Source: CAD feature listing. Evaluate the final solid. Frame: model axes, mm. Face numbers are marked on the shaded views. A direction names the side the tool comes from. Give positions to 0.01 mm unless a question says otherwise; leave off trailing zeros. Order: outer loops, then holes, each group sorted by start corner. A loop starts at its lowest first (then second) coordinate and runs counter-clockwise, first axis right, second up. Notation, with made-up numbers: (45.25, -29.75) -> (80.25, -29.75) arc R18 cw to (80.25, -7.75) -> close; hole circle Ø5 at (-9, 75.5). An arc over 180 degrees is marked (long way). Use one line per item in the form item = value. Start each with the question number.
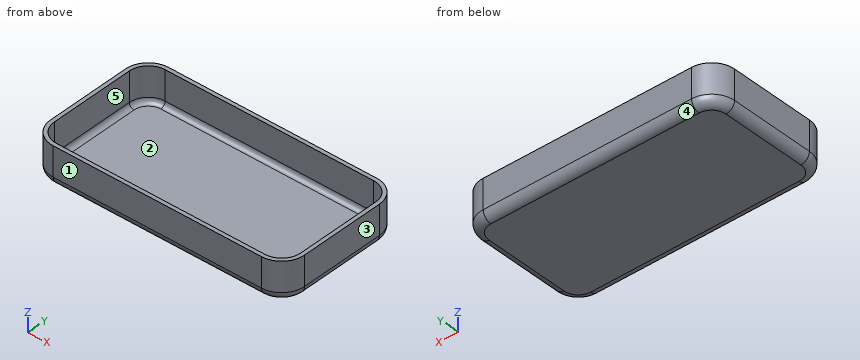
from build123d import *

# Parameters (mm, degrees)
F0_W     = 53.4
F0_H     = 27.4
F0_W_2   = 51.8
F0_H_2   = 25.8
F1_DEPTH = 0.8
F2_DEPTH = 8
F3_R     = 4
F4_R     = 4.8
F5_R     = 1
F6_R     = 1.8


with BuildPart() as f1:
    # F0 (on Top) → F1 (new body)
    with BuildSketch(Plane.XY):
        Rectangle(F0_W, F0_H)
        Rectangle(F0_W_2, F0_H_2, mode=Mode.SUBTRACT)
        Rectangle(F0_W_2, F0_H_2)
    extrude(amount=F1_DEPTH)

    # F0 (on Top) → F2 (join)
    with BuildSketch(Plane.XY):
        Rectangle(F0_W, F0_H)
        Rectangle(F0_W_2, F0_H_2, mode=Mode.SUBTRACT)
    extrude(amount=F2_DEPTH)

    # F3
    f3_edges = [f1.edges().sort_by_distance(p)[0] for p in [
        (-25.9, 12.9, 4.4),
        (25.9, 12.9, 4.4),
        (25.9, -12.9, 4.4),
        (-25.9, -12.9, 4.4),
    ]]
    fillet(f3_edges, radius=F3_R)

    # F4
    f4_edges = [f1.edges().sort_by_distance(p)[0] for p in [
        (26.7, 13.7, 4),
        (26.7, -13.7, 4),
        (-26.7, 13.7, 4),
        (-26.7, -13.7, 4),
    ]]
    fillet(f4_edges, radius=F4_R)

    # F5
    f5_edges = [f1.edges().sort_by_distance(p)[0] for p in [
        (0, 12.9, 0.8),
    ]]
    fillet(f5_edges, radius=F5_R)

    # F6
    f6_edges = [f1.edges().sort_by_distance(p)[0] for p in [
        (0, 13.7, 0),
    ]]
    fillet(f6_edges, radius=F6_R)


solid = f1.part
1) Cut plane B-B, the plane x = -8.5. Return the cut outline in (y, z).
2) Material intervals for probe 1 along Y at (x, z) = (-19, 3.25); probe 2 along X at (y, z) = (2.5, 2.25); probe 3 along Z at (x, y) = (23, 8.25), sorted ascending.
3) Cut plane A-A, the plane z = 5.5. Return the cut outline in (x, y).
4) Reachability of the marked faces 4 and 5 from +Z, -Z, +X, -X, +Y, -Y: full face, straight path, thin tool, end or side. Return the list, or none.
5) Pin query (flat end, axial travel): pin 1 (10 mm diameter, centred on x = 12.5, y = -6.5, fed in from +Z). Return the tip coordinate at first contact, or that it passes through.
6) Draft query along X for the marked faces 1, 2 and 3. Return one class per face: +X half, -X half, draft (parallel to the pull), parting line (faces both ways), or undercut.
7) Cut plane C-C, the plane y = -3.75. Return the cut outline in (x, z), plus the area to 3 significant figures.
Output values:
q1.outline = (-13.7, 1.8) arc R1.8 ccw to (-11.9, 0) -> (11.9, 0) arc R1.8 ccw to (13.7, 1.8) -> (13.7, 8) -> (12.9, 8) -> (12.9, 1.8) arc R1 cw to (11.9, 0.8) -> (-11.9, 0.8) arc R1 cw to (-12.9, 1.8) -> (-12.9, 8) -> (-13.7, 8) -> close
q2.probe_1 = -13.7 to -12.9, 12.9 to 13.7
q2.probe_2 = -26.7 to -25.9, 25.9 to 26.7
q2.probe_3 = 0 to 0.8
q3.outline = (-26.7, -8.9) arc R4.8 ccw to (-21.9, -13.7) -> (21.9, -13.7) arc R4.8 ccw to (26.7, -8.9) -> (26.7, 8.9) arc R4.8 ccw to (21.9, 13.7) -> (-21.9, 13.7) arc R4.8 ccw to (-26.7, 8.9) -> close; hole (-25.9, -8.9) arc R4 ccw to (-21.9, -12.9) -> (21.9, -12.9) arc R4 ccw to (25.9, -8.9) -> (25.9, 8.9) arc R4 ccw to (21.9, 12.9) -> (-21.9, 12.9) arc R4 ccw to (-25.9, 8.9) -> close
q4.face_4 = -Z, +X, -X, +Y
q4.face_5 = +Z
q5.pin_1 = 0.8
q6.face_1 = draft
q6.face_2 = undercut
q6.face_3 = +X half
q7.outline = (-26.7, 1.8) arc R1.8 ccw to (-24.9, 0) -> (24.9, 0) arc R1.8 ccw to (26.7, 1.8) -> (26.7, 8) -> (25.9, 8) -> (25.9, 1.8) arc R1 cw to (24.9, 0.8) -> (-24.9, 0.8) arc R1 cw to (-25.9, 1.8) -> (-25.9, 8) -> (-26.7, 8) -> close
q7.area = 53.3 mm^2
